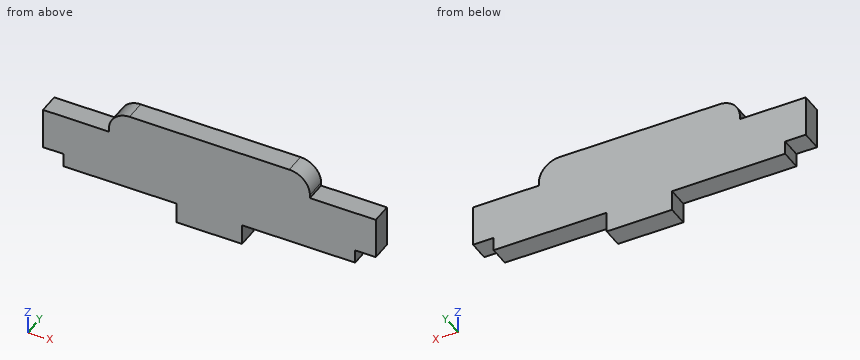
```python
from build123d import *

# Parameters (mm, degrees)
BOSS_EXTRUDE1_DEPTH = 6


with BuildPart() as part:
    # Sketch1 → Boss-Extrude1 (new body)
    with BuildSketch(Plane(origin=(0, 0, 0), x_dir=(1, 0, 0), z_dir=(0, 1, 0))):
        with BuildLine():
            Line((40.206859082, 0.405693798), (53.496778433, 0.405693798))
            Line((53.496778433, 0.405693798), (70.087810024, 0.405693798))
            ThreePointArc((70.087810024, 0.405693798), (74.330450711, 2.163053111), (76.087810024, 6.405693798))
            Line((76.087810024, 6.405693798), (76.087810024, 7.364453077))
            Line((76.087810024, 7.364453077), (95.248908352, 7.364453077))
            Line((95.248908352, 7.364453077), (95.248908352, 19.364453077))
            Line((95.248908352, 19.364453077), (89.248908352, 19.364453077))
            Line((89.248908352, 19.364453077), (89.248908352, 23.311113477))
            Line((89.248908352, 23.311113477), (56.351818757, 23.311113477))
            Line((56.351818757, 23.311113477), (56.351818757, 29.311113477))
            Line((56.351818757, 29.311113477), (37.351818757, 29.311113477))
            Line((37.351818757, 29.311113477), (37.351818757, 23.311113477))
            Line((37.351818757, 23.311113477), (4.454729162, 23.311113477))
            Line((4.454729162, 23.311113477), (4.454729162, 19.364453077))
            Line((4.454729162, 19.364453077), (-1.545270838, 19.364453077))
            Line((-1.545270838, 19.364453077), (-1.545270838, 7.364453077))
            Line((-1.545270838, 7.364453077), (17.615827491, 7.364453077))
            Line((17.615827491, 7.364453077), (17.615827491, 6.405693798))
            ThreePointArc((17.615827491, 6.405693798), (19.373186804, 2.163053111), (23.615827491, 0.405693798))
            Line((23.615827491, 0.405693798), (40.206859082, 0.405693798))
        make_face()
    extrude(amount=BOSS_EXTRUDE1_DEPTH)


solid = part.part
```
Geometry: final body of the model. Coordinates: model frame, mm. Round coordinates to 2 decimals unless told otherwise and drop trailing zeros. Order: outer loops, then holes, each group sorted by start corner. A loop starts at its lowest first (then second) coordinate and runs counter-clockwise, first axis right, second up. Notation, with made-up numbers: (74.25, 45) - (124.25, 45) arc R7 cw to (124.25, 58) - close; hole circle Ø1 at (89, 23). An arc over 180 degrees is marked (long way). Write item = value, one per line. Start each with the question number.
Q1. Cut plane A-A on y = 4.45. Return the cut outline in (x, z), and give its area (3 significant figures).
Q2. Cut plane C-C on z = -25.5. Return the cut outline in (x, y), and give its area (3 significant figures).
Q3. Cut plane B-B on x = 30. Return the cut outline in (y, z).
Q4. Pin query (flat end, axial travel): pin 1 (1.8 mm diameter, centred on x = 90.5, y = 3.5, fed in from +Z); pin 2 (1.1 mm diameter, centred on y = 2, z = -6.5, fed in from -X); pin 3 (1.8 mm diameter, centred on x = 22, y = 3.5, fed in from -Z). Return the tip coordinate at first contact, or that it passes through.
Q5. Ray query, line 1 (Z direction, x = 60.5, y = 4.45); line 2 (X direction, y = 2.7, z = -19.5); line 3 (Z direction, x = 4, y = 5.6). Return the intervals inside material, ascending. Write a range as from..to.
Outcome:
q1.outline = (-1.55, -19.36) - (4.45, -19.36) - (4.45, -23.31) - (37.35, -23.31) - (37.35, -29.31) - (56.35, -29.31) - (56.35, -23.31) - (89.25, -23.31) - (89.25, -19.36) - (95.25, -19.36) - (95.25, -7.36) - (76.09, -7.36) - (76.09, -6.41) arc R6 ccw to (70.09, -0.41) - (23.62, -0.41) arc R6 ccw to (17.62, -6.41) - (17.62, -7.36) - (-1.55, -7.36) - close
q1.area = 2,000 mm^2
q2.outline = (37.35, 0) - (56.35, 0) - (56.35, 6) - (37.35, 6) - close
q2.area = 114 mm^2
q3.outline = (0, -23.31) - (6, -23.31) - (6, -0.41) - (0, -0.41) - close
q4.pin_1 = -7.36
q4.pin_2 = 17.62
q4.pin_3 = -23.31
q5.line_1 = -23.31..-0.41
q5.line_2 = 4.45..89.25
q5.line_3 = -19.36..-7.36
